Here's the drawing with two shaded views (mm, measured from the low corner). I have some questions. A direction names the side the tool comes from. Round coordinates to 2 decimals unless told otherwise and drop trailing zeros. Write each loop counter-clockwise with the first axis right and the second up, starting at its lowest first coordinate (ties: lowest second). Pieces come first, ordered by that corner, then holes. Notation, with made-up numbers: M 42.25,28 L 81.25,28 A32 cw 81.25,66 Z; hole C -1,13.25 d8. An arc over 180 degrees is marked long. Answer as a JSON object with one key per item and string values. Group by question number.
1) Suppose I cut it at D-D, the plane y = 0.75. Write out the boundary of the cut face in (x, z).
2) I'm going to push flat-ended pins straight in: pin 1 Ø1.4 at (x, y) = (8.5, 2.5) entering from -Z; pin 2 Ø1.8 at (x, y) = (19, 2.45) entering from +Z. Where does each tip first touch, or does it pass through?
3) On a 3-axis mill with a long thin cutter (end or side, diameter ignored), from which of +Z, -Z, +X, -X, +Y, -Y can I reach the whole of each face in a straight line? I mean the marked faces 5 and 6. Say none if no direction works.
4) If we mould it in two halves opening along X, with no side actions, what happens to the marked faces 1, 2, 3 and 4? For each: +X half, -X half, draft (parallel to the pull), parting line (faces both ways), or undercut.
5) Please list where these lines run through material, in increasing order: L1, parallel to X at y = 2.4, z = 0.25; L2, parallel to X at y = 3.65, z = 0.2; L3, parallel to Y at x = 19, z = 0.3. Write a range as [from, to].
6) Suppose I cut it at B-B, the plane x = 19. Write out the boundary of the cut face in (y, z).
7) Suppose I cut it at A-A, the plane y = 2.65. State how many separate pieces and enclosed holes the cut face has.
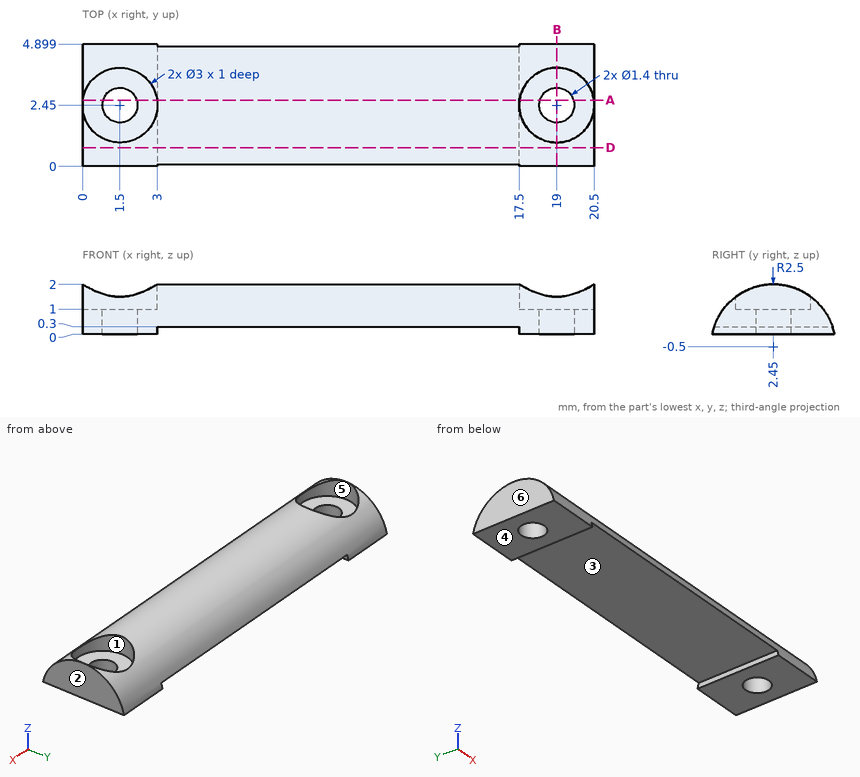
Results:
{
 "1": {"outline": "M 0,0 L 3,0 L 3,0.3 L 17.5,0.3 L 17.5,0 L 20.5,0 L 20.5,1.33 L 0,1.33 Z"},
 "2": {"pin 1": "z = 0.3", "pin 2": "z = 1"},
 "3": {"face 5": "+Z", "face 6": "+Z, -Z, -X, +Y, -Y"},
 "4": {"face 1": "undercut", "face 2": "+X half", "face 3": "undercut", "face 4": "draft"},
 "5": {"L1": "[0, 0.8], [2.2, 3], [17.5, 18.3], [19.7, 20.5]", "L2": "[0, 3], [17.5, 20.5]", "L3": "[0.08, 1.75], [3.15, 4.82]"},
 "6": {"outline": "M 0,0 L 1.75,0 L 1.75,1 L 0.95,1 L 0.95,1.5 A2.5 ccw Z; M 3.15,0 L 4.9,0 A2.5 ccw 3.95,1.5 L 3.95,1 L 3.15,1 Z"},
 "7": {"separate pieces": "3", "enclosed holes": "0"}
}
